The model under review builds one solid part; all positions refer to its coordinate system, in mm. Face numbers are marked on the shaded views. Coordinates: 2 decimals unless noted, no trailing zeros. Loops run counter-clockwise (first coordinate to the right, second up) from the corner with the lowest first, then second, coordinate; pieces in that order, holes last. Notation, with made-up numbers: M -12,27 L -7,27 A16 cw -7,47 Z; hole C 7.25,35 d6. An arc over 180 degrees is marked long. Use one line per item in the form item = value.
```python
from build123d import *

# Parameters (mm, degrees)
F0_R     = 3.3807298635
F1_DEPTH = 5


with BuildPart() as f1:
    # F0 (on Top) → F1 (new body)
    with BuildSketch(Plane.XY):
        with BuildLine():
            Line((-64.6143609347, 0), (-10, 0))
            ThreePointArc((-10, 0), (-2.9289321881, 2.9289321881), (0, 10))
            Line((0, 10), (0, 40.8130657572))
            ThreePointArc((0, 40.8130657572), (-2.9289321881, 47.8841335691), (-10, 50.8130657572))
            Line((-10, 50.8130657572), (-64.6143609347, 50.8130657572))
            ThreePointArc((-64.6143609347, 50.8130657572), (-71.6854287466, 47.8841335691), (-74.6143609347, 40.8130657572))
            Line((-74.6143609347, 40.8130657572), (-74.6143609347, 10))
            ThreePointArc((-74.6143609347, 10), (-71.6854287466, 2.9289321881), (-64.6143609347, 0))
        make_face()
        with BuildLine():
            add(Edge.make_bspline(
                [(-46.661470066, 21.0336615097), (-47.5455431911, 20.8818405408), (-48.3841733051, 20.8818405408)],
                knots=[0, 0, 0, 1, 1, 1], degree=2))
            add(Edge.make_bspline(
                [(-48.3841733051, 20.8818405408), (-50.2246152549, 20.8818405408), (-51.2408862305, 21.8340781826)],
                knots=[0, 0, 0, 1, 1, 1], degree=2))
            add(Edge.make_bspline(
                [(-51.2408862305, 21.8340781826), (-52.2571572061, 22.7863158244), (-52.2571572061, 24.4387889555)],
                knots=[0, 0, 0, 1, 1, 1], degree=2))
            add(Edge.make_bspline(
                [(-52.2571572061, 24.4387889555), (-52.2571572061, 26.0272287528), (-51.5858399966, 27.2376653213)],
                knots=[0, 0, 0, 1, 1, 1], degree=2))
            add(Edge.make_bspline(
                [(-51.5858399966, 27.2376653213), (-50.9145227871, 28.4481018898), (-49.6689711646, 29.1070255508)],
                knots=[0, 0, 0, 1, 1, 1], degree=2))
            add(Edge.make_bspline(
                [(-49.6689711646, 29.1070255508), (-48.423419542, 29.7659492119), (-46.8225861963, 29.7659492119)],
                knots=[0, 0, 0, 1, 1, 1], degree=2))
            add(Edge.make_bspline(
                [(-46.8225861963, 29.7659492119), (-45.3642786581, 29.7659492119), (-43.7696420866, 29.4292578114)],
                knots=[0, 0, 0, 1, 1, 1], degree=2))
            Line((-43.7696420866, 29.4292578114), (-44.1104646699, 27.2541900526))
            Line((-44.1104646699, 27.2541900526), (-44.6537152117, 27.2541900526))
            Line((-44.6537152117, 27.2541900526), (-44.6537152117, 28.5059384494))
            add(Edge.make_bspline(
                [(-44.6537152117, 28.5059384494), (-45.0028001606, 28.7847932903), (-45.4964765086, 28.9355814635)],
                knots=[0, 0, 0, 1, 1, 1], degree=2))
            add(Edge.make_bspline(
                [(-45.4964765086, 28.9355814635), (-45.9901528565, 29.0863696367), (-46.5313378069, 29.0863696367)],
                knots=[0, 0, 0, 1, 1, 1], degree=2))
            add(Edge.make_bspline(
                [(-46.5313378069, 29.0863696367), (-47.5971829765, 29.0863696367), (-48.4461410476, 28.4925121052)],
                knots=[0, 0, 0, 1, 1, 1], degree=2))
            add(Edge.make_bspline(
                [(-48.4461410476, 28.4925121052), (-49.2950991187, 27.8986545737), (-49.766053961, 26.8183502643)],
                knots=[0, 0, 0, 1, 1, 1], degree=2))
            add(Edge.make_bspline(
                [(-49.766053961, 26.8183502643), (-50.2370088034, 25.7380459548), (-50.2370088034, 24.3809523959)],
                knots=[0, 0, 0, 1, 1, 1], degree=2))
            add(Edge.make_bspline(
                [(-50.2370088034, 24.3809523959), (-50.2370088034, 23.0445147511), (-49.6431512719, 22.2957378636)],
                knots=[0, 0, 0, 1, 1, 1], degree=2))
            add(Edge.make_bspline(
                [(-49.6431512719, 22.2957378636), (-49.0492937404, 21.5469609761), (-47.9710550224, 21.5469609761)],
                knots=[0, 0, 0, 1, 1, 1], degree=2))
            add(Edge.make_bspline(
                [(-47.9710550224, 21.5469609761), (-47.3389840497, 21.5469609761), (-46.6996835071, 21.7318314076)],
                knots=[0, 0, 0, 1, 1, 1], degree=2))
            add(Edge.make_bspline(
                [(-46.6996835071, 21.7318314076), (-46.0603829645, 21.9167018392), (-45.6679205959, 22.1996878629)],
                knots=[0, 0, 0, 1, 1, 1], degree=2))
            Line((-45.6679205959, 22.1996878629), (-45.1701130652, 23.6208147556))
            Line((-45.1701130652, 23.6208147556), (-44.6206657491, 23.6208147556))
            Line((-44.6206657491, 23.6208147556), (-45.0482431718, 21.4250910827))
            add(Edge.make_bspline(
                [(-45.0482431718, 21.4250910827), (-45.7773969408, 21.1854824787), (-46.661470066, 21.0336615097)],
                knots=[0, 0, 0, 1, 1, 1], degree=2))
        make_face(mode=Mode.SUBTRACT)
        with BuildLine():
            add(Edge.make_bspline(
                [(-28.4233306773, 21.3889432329), (-29.2340753072, 20.8818405408), (-30.2462151, 20.8818405408)],
                knots=[0, 0, 0, 1, 1, 1], degree=2))
            add(Edge.make_bspline(
                [(-30.2462151, 20.8818405408), (-31.3430441408, 20.8818405408), (-32.0019678018, 21.5727808688)],
                knots=[0, 0, 0, 1, 1, 1], degree=2))
            add(Edge.make_bspline(
                [(-32.0019678018, 21.5727808688), (-32.6608914628, 22.2637211967), (-32.6608914628, 23.4266491627)],
                knots=[0, 0, 0, 1, 1, 1], degree=2))
            add(Edge.make_bspline(
                [(-32.6608914628, 23.4266491627), (-32.6608914628, 24.4718384181), (-32.2085269432, 25.349714769)],
                knots=[0, 0, 0, 1, 1, 1], degree=2))
            add(Edge.make_bspline(
                [(-32.2085269432, 25.349714769), (-31.7561624235, 26.2275911199), (-30.9464505893, 26.734693812)],
                knots=[0, 0, 0, 1, 1, 1], degree=2))
            add(Edge.make_bspline(
                [(-30.9464505893, 26.734693812), (-30.1367387551, 27.2417965041), (-29.1225333709, 27.2417965041)],
                knots=[0, 0, 0, 1, 1, 1], degree=2))
            add(Edge.make_bspline(
                [(-29.1225333709, 27.2417965041), (-28.0257043301, 27.2417965041), (-27.3678134648, 26.5508561762)],
                knots=[0, 0, 0, 1, 1, 1], degree=2))
            add(Edge.make_bspline(
                [(-27.3678134648, 26.5508561762), (-26.7099225995, 25.8599158482), (-26.7099225995, 24.6969878822)],
                knots=[0, 0, 0, 1, 1, 1], degree=2))
            add(Edge.make_bspline(
                [(-26.7099225995, 24.6969878822), (-26.7099225995, 23.6517986268), (-27.1612543234, 22.7739222759)],
                knots=[0, 0, 0, 1, 1, 1], degree=2))
            add(Edge.make_bspline(
                [(-27.1612543234, 22.7739222759), (-27.6125860473, 21.896045925), (-28.4233306773, 21.3889432329)],
                knots=[0, 0, 0, 1, 1, 1], degree=2))
        make_face(mode=Mode.SUBTRACT)
        with BuildLine():
            add(Edge.make_bspline(
                [(-21.2061542772, 26.8834163938), (-20.6804612624, 26.5250362835), (-20.6804612624, 25.9177524078)],
                knots=[0, 0, 0, 1, 1, 1], degree=2))
            add(Edge.make_bspline(
                [(-20.6804612624, 25.9177524078), (-20.6804612624, 25.3373212205), (-21.1059730937, 24.8467432597)],
                knots=[0, 0, 0, 1, 1, 1], degree=2))
            add(Edge.make_bspline(
                [(-21.1059730937, 24.8467432597), (-21.5314849249, 24.3561652989), (-22.3360327806, 24.0401298126)],
                knots=[0, 0, 0, 1, 1, 1], degree=2))
            add(Edge.make_bspline(
                [(-22.3360327806, 24.0401298126), (-23.1405806363, 23.7240943263), (-24.1589172033, 23.6456018526)],
                knots=[0, 0, 0, 1, 1, 1], degree=2))
            add(Edge.make_bspline(
                [(-24.1589172033, 23.6456018526), (-24.191966666, 23.5175351849), (-24.191966666, 23.2076964728)],
                knots=[0, 0, 0, 1, 1, 1], degree=2))
            add(Edge.make_bspline(
                [(-24.191966666, 23.2076964728), (-24.191966666, 21.6832900094), (-23.0228419257, 21.6832900094)],
                knots=[0, 0, 0, 1, 1, 1], degree=2))
            add(Edge.make_bspline(
                [(-23.0228419257, 21.6832900094), (-22.5456903091, 21.6832900094), (-22.1387688006, 21.8671276452)],
                knots=[0, 0, 0, 1, 1, 1], degree=2))
            add(Edge.make_bspline(
                [(-22.1387688006, 21.8671276452), (-21.7318472921, 22.0509652811), (-21.3765655689, 22.2905738851)],
                knots=[0, 0, 0, 1, 1, 1], degree=2))
            Line((-21.3765655689, 22.2905738851), (-21.0935795452, 21.8836523765))
            add(Edge.make_bspline(
                [(-21.0935795452, 21.8836523765), (-21.661617184, 21.4065007599), (-22.3267376192, 21.1441706504)],
                knots=[0, 0, 0, 1, 1, 1], degree=2))
            add(Edge.make_bspline(
                [(-22.3267376192, 21.1441706504), (-22.9918580545, 20.8818405408), (-23.6053387044, 20.8818405408)],
                knots=[0, 0, 0, 1, 1, 1], degree=2))
            add(Edge.make_bspline(
                [(-23.6053387044, 20.8818405408), (-24.7476107563, 20.8818405408), (-25.347665062, 21.4571077496)],
                knots=[0, 0, 0, 1, 1, 1], degree=2))
            add(Edge.make_bspline(
                [(-25.347665062, 21.4571077496), (-25.9477193678, 22.0323749583), (-25.9477193678, 23.1426303433)],
                knots=[0, 0, 0, 1, 1, 1], degree=2))
            add(Edge.make_bspline(
                [(-25.9477193678, 23.1426303433), (-25.9477193678, 24.2528857282), (-25.4767645254, 25.2020249829)],
                knots=[0, 0, 0, 1, 1, 1], degree=2))
            add(Edge.make_bspline(
                [(-25.4767645254, 25.2020249829), (-25.005809683, 26.1511642376), (-24.2312129028, 26.6964803709)],
                knots=[0, 0, 0, 1, 1, 1], degree=2))
            add(Edge.make_bspline(
                [(-24.2312129028, 26.6964803709), (-23.4566161226, 27.2417965041), (-22.6241827828, 27.2417965041)],
                knots=[0, 0, 0, 1, 1, 1], degree=2))
            add(Edge.make_bspline(
                [(-22.6241827828, 27.2417965041), (-21.7318472921, 27.2417965041), (-21.2061542772, 26.8834163938)],
                knots=[0, 0, 0, 1, 1, 1], degree=2))
        make_face(mode=Mode.SUBTRACT)
        with BuildLine():
            Line((-41.0327334632, 26.1635577861), (-41.0761108829, 25.9755889674))
            add(Edge.make_bspline(
                [(-41.0761108829, 25.9755889674), (-40.0825614128, 27.2417965041), (-38.6118603262, 27.2417965041)],
                knots=[0, 0, 0, 1, 1, 1], degree=2))
            add(Edge.make_bspline(
                [(-38.6118603262, 27.2417965041), (-37.9859861278, 27.2417965041), (-37.6048845119, 26.8958099423)],
                knots=[0, 0, 0, 1, 1, 1], degree=2))
            add(Edge.make_bspline(
                [(-37.6048845119, 26.8958099423), (-37.223782896, 26.5498233805), (-37.223782896, 25.9569986447)],
                knots=[0, 0, 0, 1, 1, 1], degree=2))
            add(Edge.make_bspline(
                [(-37.223782896, 25.9569986447), (-37.223782896, 25.6203072442), (-37.333259241, 25.0212857342)],
                knots=[0, 0, 0, 1, 1, 1], degree=2))
            Line((-37.333259241, 25.0212857342), (-37.9467398909, 21.5924039872))
            Line((-37.9467398909, 21.5924039872), (-37.1969302077, 21.4374846312))
            Line((-37.1969302077, 21.4374846312), (-37.2816194556, 21.0119727999))
            Line((-37.2816194556, 21.0119727999), (-39.7727227007, 21.0119727999))
            Line((-39.7727227007, 21.0119727999), (-39.1137990397, 24.6845943337))
            add(Edge.make_bspline(
                [(-39.1137990397, 24.6845943337), (-38.9733388236, 25.434404017), (-38.9733388236, 25.6926029437)],
                knots=[0, 0, 0, 1, 1, 1], degree=2))
            add(Edge.make_bspline(
                [(-38.9733388236, 25.6926029437), (-38.9733388236, 26.3184771421), (-39.5599667851, 26.3184771421)],
                knots=[0, 0, 0, 1, 1, 1], degree=2))
            add(Edge.make_bspline(
                [(-39.5599667851, 26.3184771421), (-39.9668882936, 26.3184771421), (-40.4770893729, 25.8661126225)],
                knots=[0, 0, 0, 1, 1, 1], degree=2))
            add(Edge.make_bspline(
                [(-40.4770893729, 25.8661126225), (-40.9872904521, 25.4137481028), (-41.2310302389, 24.845710464)],
                knots=[0, 0, 0, 1, 1, 1], degree=2))
            Line((-41.2310302389, 24.845710464), (-41.9168065883, 21.0119727999))
            Line((-41.9168065883, 21.0119727999), (-43.6333130533, 21.0119727999))
            Line((-43.6333130533, 21.0119727999), (-42.1233657297, 29.6027674902))
            Line((-42.1233657297, 29.6027674902), (-42.7099936913, 29.7576868462))
            Line((-42.7099936913, 29.7576868462), (-42.6397635832, 30.1852642689))
            Line((-42.6397635832, 30.1852642689), (-40.28292378, 30.1852642689))
            Line((-40.28292378, 30.1852642689), (-40.8261743218, 27.196353493))
            Line((-40.8261743218, 27.196353493), (-41.0327334632, 26.1635577861))
        make_face(mode=Mode.SUBTRACT)
        Polygon((-32.8860409269, 30.1852642689), (-34.4104473904, 21.5924039872), (-33.6420473844, 21.4374846312), (-33.7122774925, 21.0119727999), (-36.2488237487, 21.0119727999), (-34.7264828767, 29.6027674902), (-35.3131108382, 29.7576868462), (-35.2428807301, 30.1852642689), align=None, mode=Mode.SUBTRACT)
        with Locations((-10, 40.8130657572)):
            Circle(F0_R, mode=Mode.SUBTRACT)
    extrude(amount=F1_DEPTH)


solid = f1.part
```
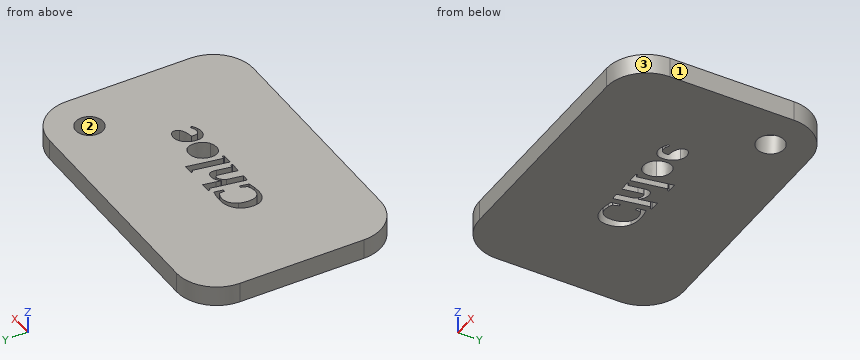
1. Wall thickness on line 1 along Y through (x, z) = (-10, 2.4); line 2 along X through (y, z) = (9.5, 4.65); line 3 along Y through (x, z) = (-27, 4.6): over which ranges is each line inside the solid? List them lowest first. Write a range as from..to.
Response values:
line_1 = 0..37.43, 44.19..50.81
line_2 = -74.6..-0.01
line_3 = 0..23.13, 26.03..50.81
2. Add section B-B (z = 1.2). Count the separate pieces of the cut face and the enclosed holes in it, then the cut area to 3 significant figures.
Response values:
separate_pieces = 1
enclosed_holes = 6
area = 3,550 mm^2
3. Insertion check: P1, Ø2, axis at y = 42.5, z = 3.5, coming from the +X side. The pin has a flat end and moves straight along its axis. Give the tip position at first contact, or say it passes through.
Response values:
P1 = -0.02
4. The part is to be moulded in two halves that separate along Y. For the marked faces 1, 2 and 3, say which applies: pulls with the +Y half, pulls with the -Y half, needs draft (parallel to the pull), parting line crosses it, or undercut.
Response values:
face_1 = needs draft
face_2 = undercut
face_3 = pulls with the -Y half
5. Add section A-A (y = 39). State the section outline as (x, z) points.
Response values:
outline = M -74.61,0 L -12.85,0 L -12.85,5 L -74.61,5 Z; M -7.15,0 L 0,0 L 0,5 L -7.15,5 Z
